Source: CAD feature listing. Evaluate the final solid. Frame: model axes, mm. Face numbers are marked on the shaded views. Round coordinates to 2 decimals unless told otherwise and drop trailing zeros. Loops run counter-clockwise (first coordinate to the right, second up) from the corner with the lowest first, then second, coordinate; pieces in that order, holes last. Notation, with made-up numbers: (10.25, -4) - (17.25, -4) arc R21 ccw to (17.25, 11) - close; hole circle Ø9 at (52.5, 23). An arc over 180 degrees is marked (long way). One line per question, with ' | ' between items. Start each with the question number.
1. Cut plane D-D (y = -3.75). Return loops of the section in (x, z).
2. Cut plane C-C (z = 4.3). Return loops of the section in (x, y).
3. Mould query, pull axis Y, two halves, no side actions, for the marked faces 1, 2, 3 and 4. Classes: pulls with the +Y half, pulls with the -Y half, needs draft (parallel to the pull), parting line crosses it, or undercut.
4. Pin query (flat end, axial travel): pin 1 (1.5 mm diameter, centred on x = -12.5, z = 2, fed in from -Y); pin 2 (3 mm diameter, centred on x = -18.46, y = -4.3, fed in from -Z); pin 3 (1.5 mm diameter, centred on x = -27, z = 2.5, fed in from +Y). Return the tip coordinate at first contact, or that it passes through.
5. Cut plane B-B (x = -24). Return loops of the section in (y, z), then the cut area to 3 significant figures.
6. Ray query, line 1 (X direction, y = 6.75, z = 3.75); line 2 (X direction, y = -4, z = 2.05); line 3 (Y direction, x = -17.5, z = 1.65). Return the intervals inside material, ascending.
7. Cut plane A-A (y = 7.5). Return loops of the section in (x, z).
```python
from build123d import *

# Parameters (mm, degrees)
ESQUISSE1_R        = 1.8
BOSS_EXTRU_1_DEPTH = 5
CONG_1_R           = 4


with BuildPart() as part:
    # Esquisse1 → Boss.-Extru.1 (new body)
    with BuildSketch(Plane.XY):
        Polygon((-32.799356044, 12.280796054), (-2.817383551, 11.058367683), (-18.866700046, -14.287626874), align=None)
        with Locations((-18.459525699, -4.301037602)):
            Circle(ESQUISSE1_R, mode=Mode.SUBTRACT)
        with Locations((-24.365403682, 6.945977976)):
            Circle(ESQUISSE1_R, mode=Mode.SUBTRACT)
        with Locations((-11.657643474, 6.427855741)):
            Circle(ESQUISSE1_R, mode=Mode.SUBTRACT)
    extrude(amount=BOSS_EXTRU_1_DEPTH)

    # Congé1
    cong_1_edges = [part.edges().sort_by_distance(p)[0] for p in [
        (-32.799356044, 12.280796054, 2.5),
        (-2.817383551, 11.058367683, 2.5),
        (-18.866700046, -14.287626874, 2.5),
    ]]
    fillet(cong_1_edges, radius=CONG_1_R)


solid = part.part
```
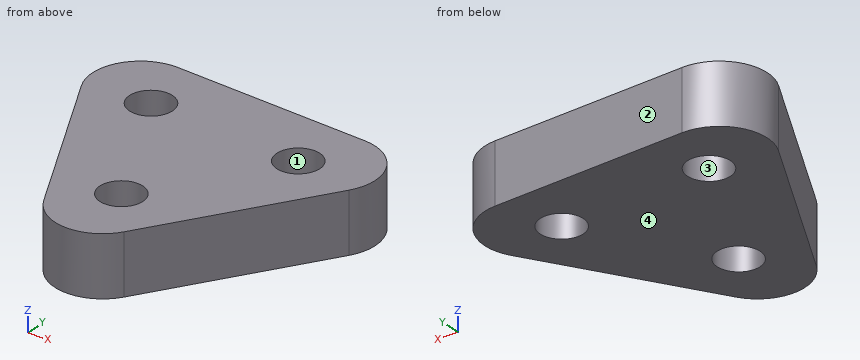
Answers follow:
1) outline: (-24.39, 0) - (-20.17, 0) - (-20.17, 5) - (-24.39, 5) - close; (-16.75, 0) - (-12.19, 0) - (-12.19, 5) - (-16.75, 5) - close
2) outline: (-29.58, 6.14) - (-22.08, -8.15) arc R4 ccw to (-15.16, -8.44) - (-6.52, 5.2) arc R4 ccw to (-9.74, 11.34) - (-25.88, 12) arc R4 ccw to start; hole circle Ø3.6 at (-24.37, 6.95); hole circle Ø3.6 at (-18.46, -4.3); hole circle Ø3.6 at (-11.66, 6.43)
3) face 1: undercut | face 2: pulls with the +Y half | face 3: undercut | face 4: needs draft
4) pin 1: stops at y = -5.42 | pin 2: passes through | pin 3: stops at y = 12
5) outline: (-4.5, 0) - (5.18, 0) - (5.18, 5) - (-4.5, 5) - close; (8.71, 0) - (11.92, 0) - (11.92, 5) - (8.71, 5) - close | area: 64.5 mm2
6) line 1: x = -29.84 to -26.15, -22.58 to -13.43, -9.89 to -5.95 | line 2: x = -24.26 to -20.23, -16.68 to -12.35 | line 3: y = -10.16 to -5.82, -2.78 to 11.66
7) outline: (-30.01, 0) - (-26.08, 0) - (-26.08, 5) - (-30.01, 5) - close; (-22.65, 0) - (-13.1, 0) - (-13.1, 5) - (-22.65, 5) - close; (-10.21, 0) - (-5.91, 0) - (-5.91, 5) - (-10.21, 5) - close
